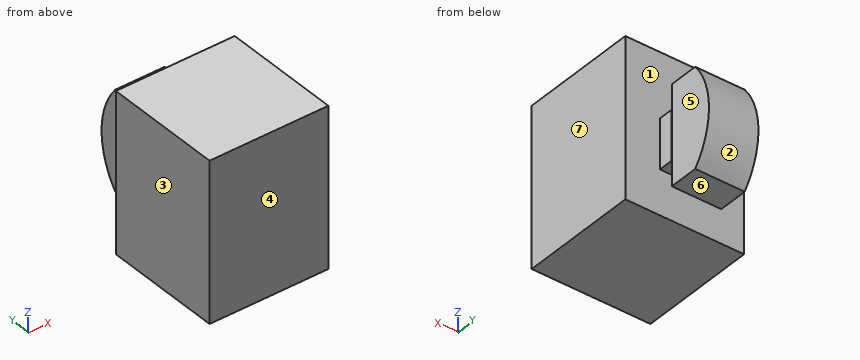
```python
from build123d import *

# Parameters (mm, degrees)
SKETCH_1_W      = 12
SKETCH_1_H      = 12
EXTRUDE_1_DEPTH = 16
SKETCH_2_W      = 5
SKETCH_2_H      = 5
EXTRUDE_2_DEPTH = 1.5
SKETCH_3_W      = 5
SKETCH_3_H      = 10
EXTRUDE_3_DEPTH = 3
EXTRUDE_4_DEPTH = 5


with BuildPart() as part:
    # 스케치1 → 보스-돌출1 (new body)
    with BuildSketch(Plane.XY):
        Rectangle(SKETCH_1_W, SKETCH_1_H)
    extrude(amount=EXTRUDE_1_DEPTH)

    # 스케치2 → 보스-돌출2 (add)
    with BuildSketch(Plane(origin=(0, 6, 0), x_dir=(1, 0, 0), z_dir=(0, 1, 0))):
        with Locations((0, -7)):
            Rectangle(SKETCH_2_W, SKETCH_2_H)
    extrude(amount=EXTRUDE_2_DEPTH)

    # 스케치3 → 보스-돌출3 (add)
    with BuildSketch(Plane(origin=(0, 7.5, 0), x_dir=(1, 0, 0), z_dir=(0, 1, 0))):
        with Locations((-0.014967469, -7)):
            Rectangle(SKETCH_3_W, SKETCH_3_H)
    extrude(amount=EXTRUDE_3_DEPTH)

    # 스케치4 → 보스-돌출4 (add)
    with BuildSketch(Plane.ZY.offset(2.514967469)):
        with BuildLine():
            Line((2, 10.5), (12, 10.5))
            ThreePointArc((12, 10.5), (7, 12.255002002), (2, 10.5))
        make_face()
    extrude(amount=-EXTRUDE_4_DEPTH)


solid = part.part
```
Geometry: final body of the model. Coordinates: model frame, mm. Face numbers are marked on the shaded views. A direction names the side the tool comes from. Coordinates: 2 decimals unless noted, no trailing zeros. Order: outer loops, then holes, each group sorted by start corner. A loop starts at its lowest first (then second) coordinate and runs counter-clockwise, first axis right, second up. Notation, with made-up numbers: M -24.5,-20.75 L 10.5,-20.75 A31 cw 10.5,9.25 Z; hole C 72,77 d3. An arc over 180 degrees is marked long. Answer as CSV lines item,"result".
Q1. Section B-B on z = 7. Return the cut outline in (x, y) (3 decimals), and give its area (3 significant figures).
Answers:
outline,"M -6,-6 L 6,-6 L 6,6 L 2.5,6 L 2.5,7.5 L 2.485,7.5 L 2.485,12.255 L -2.515,12.255 L -2.515,7.5 L -2.5,7.5 L -2.5,6 L -6,6 Z"
area,"175 mm^2"
Q2. Section C-C on z = 3. Return the cut outline in (x, y).
Answers:
outline,"M -6,-6 L 6,-6 L 6,6 L -6,6 Z; M -2.51,7.5 L 2.49,7.5 L 2.49,11.18 L -2.51,11.18 Z"
Q3. Section D-D on y = 7.75. Return the cut outline in (x, z), and give its area (3 significant figures).
Answers:
outline,"M -2.51,2 L 2.49,2 L 2.49,12 L -2.51,12 Z"
area,"50.0 mm^2"
Q4. Section A-A on x = 2.25. Return the cut outline in (y, z) (3 decimals).
Answers:
outline,"M -6,0 L 6,0 L 6,4.5 L 7.5,4.5 L 7.5,2 L 10.5,2 A8 ccw 10.5,12 L 7.5,12 L 7.5,9.5 L 6,9.5 L 6,16 L -6,16 Z"
Q5. Set-up query: the marked faces 5, 6 and 7. Return all of +Z, -Z, +X, -X, +Y, -Y with unobstructed straight access to the full face (end or side cutting, diameter ignored); none if empty.
Answers:
face 5,"+Z, -Z, +X, +Y"
face 6,"-Z, +X, -X, +Y"
face 7,"+Z, -Z, +X, +Y, -Y"
Q6. Line query: probe 1 along Y at (x, z) = (2.75, 4.25); probe 2 along Z at (x, y) = (1.5, 8.5); probe 3 along Y at (x, z) = (0.75, 10.5). Output: solid intervals per line, ascending. Write a range as [from, to].
Answers:
probe 1,"y = [-6, 6]"
probe 2,"z = [2, 12]"
probe 3,"y = [-6, 6], [7.5, 11.45]"
Q7. Draft query along Y for the marked faces 1, 2, 3 and 4. Return one class per face: pulls with the +Y half, pulls with the -Y half, needs draft (parallel to the pull), parting line crosses it, or undercut.
Answers:
face 1,"undercut"
face 2,"pulls with the +Y half"
face 3,"needs draft"
face 4,"pulls with the -Y half"
Q8. First-contact query: P1, Ø1.6, axis at y = 7, z = 6.5, coming from the +X side; P2, Ø2, axis at x = -4, y = 8, coming from the +Z side; P3, Ø2.5, axis at x = 0.5, y = 9.5, coming from the +Z side; P4, Ø0.8, axis at x = 0, y = 6.5, coming from the -Z side. Flat tips, straight axial feed; report the tip coordinate or a pass-through.
Answers:
P1,"stops at x = 2.5"
P2,"passes through"
P3,"stops at z = 12"
P4,"stops at z = 4.5"
